```python
from build123d import *

# Parameters (mm, degrees)
F1_DEPTH = 12.7
F3_D     = 6.35
F3_DEPTH = 12.7
F3_TIP   = 1.9077324654


# Not quite as in the source:
# - a feature names something its author has since deleted; it is built from what else it names


with BuildPart() as f1:
    # F0 (on Top) → F1 (new body, symmetric)
    with BuildSketch(Plane.XY):
        Polygon((36.83, -12.7), (36.83, 12.7), (-36.83, 12.7), (-36.83, -12.7), (-35.56, -12.7), (-35.56, 11.43), (35.56, 11.43), (35.56, -12.7), align=None)
    extrude(amount=F1_DEPTH, both=True)

    # F3
    with Locations(Plane.XZ.offset(-11.43)):
        with Locations((0, 0)):
            Hole(F3_D / 2, depth=F3_DEPTH)
            with Locations((0, 0, -(F3_DEPTH + F3_TIP / 2))):  # 118° drill point
                Cone(0, F3_D / 2, F3_TIP, mode=Mode.SUBTRACT)


solid = f1.part
```
Verification items for the finished model (mm, model axes). A direction names the side the tool comes from. Give positions to 0.01 mm unless a question says otherwise; leave off trailing zeros. Order: outer loops, then holes, each group sorted by start corner. A loop starts at its lowest first (then second) coordinate and runs counter-clockwise, first axis right, second up. Notation, with made-up numbers: (-12, 10.25) - (43, 10.25) arc R8 ccw to (43, 16.25) - close; hole circle Ø9 at (-23.5, 37). An arc over 180 degrees is marked (long way). Answer as CSV lines item,"result". Start each with the question number.
Item 1: Section check D-D, the plane z = 7.5. Record the boundary of the cut face in (x, y).
Item 2: Mould release check, pull along X, two halves, no side actions. Record for faces 3 (the face through (-36, -12.7, 0)), 4 (the face through (0.69, 12.07, -3.1)), 5 (the face through (36.83, 0, 0)), 6 (the face through (-36.83, 0, 0)): released by +X, released by -X, zero draft, split by the parting line, or undercut.
Item 3: Access from +Z, -Z, +X, -X, +Y, -Y to the whole of each face (thin tool, end or side, straight path). Record for faces 1 (the face through (0, 11.43, -5)), 2 (the face through (-17, 12, 12.7)).
Item 4: Section check A-A, the plane x = 0. Record the boundary of the cut face in (y, z) (3 decimals), plus the area to 3 significant figures.
Item 5: Material ranges on L1, parallel to Z at x = 0, y = 12.1 (3 decimals); L2, parallel to X at y = 1.5, z = -10.5; L3, parallel to Y at x = -25, z = -0.25, recorded low to high.
Item 6: Section check C-C, the plane y = -1.5. Record the boundary of the cut face in (x, z).
Item 7: Section check B-B, the plane z = 0. Record the boundary of the cut face in (x, y) (3 decimals).
Filled in:
1,outline,"(-36.83, -12.7) - (-35.56, -12.7) - (-35.56, 11.43) - (35.56, 11.43) - (35.56, -12.7) - (36.83, -12.7) - (36.83, 12.7) - (-36.83, 12.7) - close"
2,face 3,"zero draft"
2,face 4,"undercut"
2,face 5,"released by +X"
2,face 6,"released by -X"
3,face 1,"+Z, -Z, -Y"
3,face 2,"+Z, +X, -X, +Y, -Y"
4,outline,"(11.43, -12.7) - (12.7, -12.7) - (12.7, -3.175) - (11.43, -3.175) - close; (11.43, 3.175) - (12.7, 3.175) - (12.7, 12.7) - (11.43, 12.7) - close"
4,area,"24.2 mm^2"
5,L1,"-12.7 to -3.175, 3.175 to 12.7"
5,L2,"-36.83 to -35.56, 35.56 to 36.83"
5,L3,"11.43 to 12.7"
6,outline,"(-36.83, -12.7) - (-35.56, -12.7) - (-35.56, 12.7) - (-36.83, 12.7) - close; (35.56, -12.7) - (36.83, -12.7) - (36.83, 12.7) - (35.56, 12.7) - close"
7,outline,"(-36.83, -12.7) - (-35.56, -12.7) - (-35.56, 11.43) - (-3.175, 11.43) - (-3.175, 12.7) - (-36.83, 12.7) - close; (3.175, 11.43) - (35.56, 11.43) - (35.56, -12.7) - (36.83, -12.7) - (36.83, 12.7) - (3.175, 12.7) - close"
